from build123d import *

# Parameters (mm, degrees)
SWEEP5_PROFILE_R = 0.95
SWEEP6_PROFILE_R = 0.95
SWEEP7_PROFILE_R = 0.95


with BuildPart() as part:
    # Sweep5: sweep along a path in Sketch1
    with BuildLine(Plane.XY) as sweep5_path:
        Line((0, 0), (0, 4))
        ThreePointArc((0, 4), (0.585786438, 5.414213562), (2, 6))
        Line((2, 6), (12, 6))
        ThreePointArc((12, 6), (13.414213562, 5.414213562), (14, 4))
        Line((14, 4), (14, 0))
    # Sweep5 profile (on start of the path) → Sweep5 (sweep)
    with BuildSketch(Plane.ZX):
        Circle(SWEEP5_PROFILE_R)
    sweep(path=sweep5_path.line)

    # Sweep6: sweep along a path in Sketch3
    with BuildLine(Plane(origin=(14, 0, 0), x_dir=(0, -1, 0), z_dir=(-1, 0, 0))) as sweep6_path:
        Line((1, 11), (1, 1))
        ThreePointArc((1, 1), (0.707106781, 0.292893219), (0, 0))
    # Sweep6 profile (on start of the path) → Sweep6 (sweep)
    with BuildSketch(Plane(origin=(14, -1, 11), x_dir=(0, -1, 0), z_dir=(0, 0, -1))):
        Circle(SWEEP6_PROFILE_R)
    sweep(path=sweep6_path.line)

    # Sweep7: sweep along a path in Sketch2
    with BuildLine(Plane(origin=(0, 0, 0), x_dir=(0, 0, -1), z_dir=(1, 0, 0))) as sweep7_path:
        Line((-11, -1), (-1, -1))
        ThreePointArc((-1, -1), (-0.292893219, -0.707106781), (0, 0))
    # Sweep7 profile (on start of the path) → Sweep7 (sweep)
    with BuildSketch(Plane(origin=(0, -1, 11), x_dir=(0, -1, 0), z_dir=(0, 0, -1))):
        Circle(SWEEP7_PROFILE_R)
    sweep(path=sweep7_path.line)


solid = part.part
The listing builds one solid part. Answer for the finished solid, in the listing's coordinates (mm). A direction names the side the tool comes from. Coordinates: 2 decimals unless noted, no trailing zeros. Order: outer loops, then holes, each group sorted by start corner. A loop starts at its lowest first (then second) coordinate and runs counter-clockwise, first axis right, second up. Notation, with made-up numbers: (-22, -5) -> (-15, -5) arc R14 ccw to (-15, 5) -> close; hole circle Ø1 at (87, 57). An arc over 180 degrees is marked (long way). Answer in a Markdown table with one row per item. Add a question column.
Item 1: Each of these flat-tipped pins is pushed along its axis until it touches: P1, Ø1, axis at x = 1, z = 7, coming from the +Y side; P2, Ø2, axis at x = 9, y = 4, coming from the -Z side; P3, Ø4, axis at x = 11, z = 0.5, coming from the +Y side; P4, Ø5, axis at x = 9.5, z = 3, coming from the -Y side. Where does it stop, or does it pass through?
Item 2: Determine the mould class of faces 4 (the face through (0, -1, 11)), 5 (the face through (13.058, -0.876, 5.93)) for opening direction X: +X half, -X half, draft (parallel to the pull), parting line (faces both ways), or undercut.
Item 3: Find section B-B (z = 2.5). Write down the section's boundary in (x, y), then the cut area to 3 significant figures.
Item 4: Which of the six approach directions +Z, -Z, +X, -X, +Y, -Y give full straight-line access (tool end or side, diameter ignored) to faces 1 (the face through (14, -1, 11)), 2 (the face through (-0.3, -1.9, 5.9)), 3 (the face through (13.058, 1.972, -0.124))?
Item 5: Find section C-C (x = 10.25). Write down the section's boundary in (y, z), then the cut area to 3 significant figures.
Item 6: Find section A-A (y = 1.75). Write down the section's boundary in (x, z).
Item 7: Find the intervals of material crossed by L1, parallel to X at y = -1, z = 5.5; L2, parallel to Z at x = 0.75, y = 6; L3, parallel to Z at x = 8.5, y = 6.75, in increasing order. Write a range as from..to.
Result set:
| question | item | result |
|---|---|---|
| 1 | P1 | stops at y = -0.19 |
| 1 | P2 | passes through |
| 1 | P3 | stops at y = 6.95 |
| 1 | P4 | stops at y = 5.19 |
| 2 | face 4 | draft |
| 2 | face 5 | undercut |
| 3 | outline | circle Ø1.9 at (0, -1); circle Ø1.9 at (14, -1) |
| 3 | area | 5.67 mm² |
| 4 | face 1 | +Z, +X, -X, +Y, -Y |
| 4 | face 2 | +Z |
| 4 | face 3 | none |
| 5 | outline | circle Ø1.9 at (6, 0) |
| 5 | area | 2.84 mm² |
| 6 | outline | circle Ø1.9 at (0, 0); circle Ø1.9 at (14, 0) |
| 7 | L1 | x = -0.95..0.95, 13.05..14.95 |
| 7 | L2 | z = -0.88..0.88 |
| 7 | L3 | z = -0.58..0.58 |
